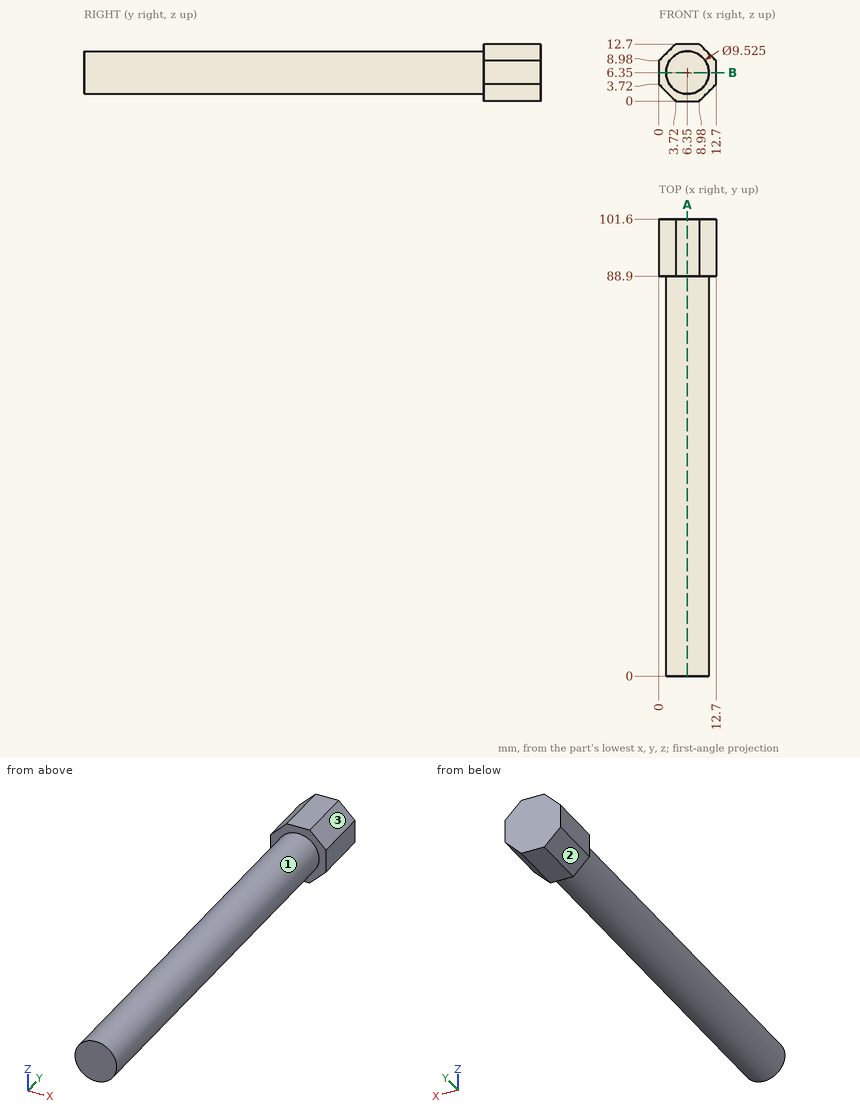
Drawing for the job (mm, zero at the part's lowest x, y, z). Give positions to 0.01 mm unless a question says otherwise; leave off trailing zeros. Loops run counter-clockwise (first coordinate to the right, second up) from the corner with the lowest first, then second, coordinate; pieces in that order, holes last. Notation, with made-up numbers: (77.5, -8.5) - (87.5, -8.5) arc R26 ccw to (87.5, 10.5) - close; hole circle Ø6 at (-13.75, 74). An arc over 180 degrees is marked (long way). Write item = value, one per line. Start each with the question number.
1) Drop a flat-ended pin along its axis: pin 1 Ø1 at (x, y) = (6.5, 20.5) entering from -Z. Give the stop position or say it passes through.
2) Band-saw the part on B-B on z = 6.35. Give the cut face in (x, y).
3) Probe probe 1 along Y at (x, z) = (1, 9.25); probe 2 along Z at (x, y) = (6.5, 70.5); probe 3 along X at (y, z) = (55.5, 10). List the from-to ranges inside material, lowest first. Write a range as from..to.
4) Band-saw the part on A-A on x = 6.35. Give the cut face in (y, z), plus the area to 3 significant figures.
5) Pull direction Z, two halves, no side cores. Call the marked faces 1, 2 and 3: +Z half, -Z half, draft (parallel to the pull), parting line (faces both ways), or undercut.
Final values:
q1.pin_1 = 1.59
q2.outline = (0, 88.9) - (1.59, 88.9) - (1.59, 0) - (11.11, 0) - (11.11, 88.9) - (12.7, 88.9) - (12.7, 101.6) - (0, 101.6) - close
q3.probe_1 = 88.9..101.6
q3.probe_2 = 1.59..11.11
q3.probe_3 = 3.29..9.41
q4.outline = (0, 1.59) - (88.9, 1.59) - (88.9, 0) - (101.6, 0) - (101.6, 12.7) - (88.9, 12.7) - (88.9, 11.11) - (0, 11.11) - close
q4.area = 1,010 mm²
q5.face_1 = parting line
q5.face_2 = -Z half
q5.face_3 = +Z half
